```python
from build123d import *

# Parameters (mm, degrees)
CYLINDER013_R                      = 2.5
CYLINDER013_DEPTH                  = 19
CYLINDER012_R                      = 4.36
CYLINDER012_DEPTH                  = 5
FUSION001018017017_PLACEMENT_ANGLE = 180
POCKET002018_DEPTH                 = 2.5


with BuildPart() as cylinder013:
    # Cylinder013 → Cylinder013 (new body)
    with BuildSketch(Plane.XY):
        Circle(CYLINDER013_R)
    extrude(amount=CYLINDER013_DEPTH)


with BuildPart() as obj1:
    # Cylinder012 → Cylinder012 (new body)
    with BuildSketch(Plane.XY):
        Circle(CYLINDER012_R)
    extrude(amount=CYLINDER012_DEPTH)

    # Fusion001018017017: union Cylinder013
    add(cylinder013.part)


with BuildPart() as obj1_1:
    # Fusion001018017017 placement: moved
    add(obj1.part.rotate(Axis((0, 0, 0), (0, 1, 0)), FUSION001018017017_PLACEMENT_ANGLE))

    # Sketch019 → Pocket002018 (cut)
    with BuildSketch(Plane(origin=(0, 0, 0), x_dir=(-1, 0, 0), z_dir=(0, 0, 1))):
        Polygon((2, -1.154701), (2, 1.154701), (0, 2.309401), (-2, 1.154701), (-2, -1.154701), (0, -2.309401), align=None)
    extrude(amount=-POCKET002018_DEPTH, mode=Mode.SUBTRACT)


solid = obj1_1.part
```
Can you work these out from the model? Positions are in its coordinate system, mm. A direction names the side the tool comes from. Give positions to 0.01 mm unless a question says otherwise; leave off trailing zeros. Order: outer loops, then holes, each group sorted by start corner. A loop starts at its lowest first (then second) coordinate and runs counter-clockwise, first axis right, second up. Notation, with made-up numbers: (15.5, 88.5) - (61.5, 88.5) arc R11 cw to (61.5, 99.5) - close; hole circle Ø8 at (23, 31.5). An arc over 180 degrees is marked (long way). Use a Markdown table: item, result. Add a question column.
Q1. On a 3-axis mill with a long thin cutter (end or side, diameter ignored), from which of +Z, -Z, +X, -X, +Y, -Y can I reach the whole of each face in a straight line? I mean faces 1 (the flat face through (-2, -2, -5)), 2 (the flat face through (-0.99, 1.74, -1.23)), 3 (the cylindrical face through (0.945, -4.256, -2.465)). Say none if no direction works.
Q2. If we section it at B-B on y = 0: Write out the boundary of the cut face in (x, z).
Q3. If we section it at C-C on x = 1.5: Write out the boundary of the cut face in (y, z).
Q4. If we section it at A-A on z = -1.5: Write out the boundary of the cut face in (x, y), plus the area to 3 significant figures.
Q5. If we mould it in two halves opening along Y, with no side actions, what happens to faces 4 (the cylindrical face through (0.54, -2.44, -11.9)), 5 (the flat face through (-1, -2, 0)), 6 (the flat face through (-1.014, -1.724, -1.232))? For each: released by +Y, released by -Y, zero draft, split by the parting line, or undercut.
Q6. I'm going to push flat-ended pins straight in: pin 1 (2 mm diameter, centred on x = 0.5, y = 1, fed in from +Z); pin 2 (5 mm diameter, centred on y = -0.5, z = -15, fed in from +X); pin 3 (1.5 mm diameter, centred on y = -2, z = -3, fed in from -X); pin 4 (5 mm diameter, centred on y = -3, z = -12, fed in from +X). Where does each tip first touch, or does it pass through?
Q7. Please list where these lines run through material, in increasing order: line 1 along Z through (x, y) = (2.5, -3); line 2 along Z through (x, y) = (-0.75, -1); line 3 along X through (y, z) = (0, -7.25).
Q8. If we section it at D-D on z = -8.5: Write out the boundary of the cut face in (x, y), plus the area to 3 significant figures.
Answers follow:
| question | item | result |
|---|---|---|
| 1 | face 1 | -Z |
| 1 | face 2 | +Z |
| 1 | face 3 | +Z, -Z |
| 2 | outline | (-4.36, -5) - (-2.5, -5) - (-2.5, -19) - (2.5, -19) - (2.5, -5) - (4.36, -5) - (4.36, 0) - (2, 0) - (2, -2.5) - (-2, -2.5) - (-2, 0) - (-4.36, 0) - close |
| 3 | outline | (-4.09, -5) - (-2, -5) - (-2, -19) - (2, -19) - (2, -5) - (4.09, -5) - (4.09, 0) - (1.44, 0) - (1.44, -2.5) - (-1.44, -2.5) - (-1.44, 0) - (-4.09, 0) - close |
| 4 | outline | circle Ø8.72 at (0, 0); hole (-2, -1.15) - (0, -2.31) - (2, -1.15) - (2, 1.15) - (0, 2.31) - (-2, 1.15) - close |
| 4 | area | 45.9 mm^2 |
| 5 | face 4 | split by the parting line |
| 5 | face 5 | zero draft |
| 5 | face 6 | undercut |
| 6 | pin 1 | stops at z = 0 |
| 6 | pin 2 | stops at x = 2.5 |
| 6 | pin 3 | stops at x = -4.18 |
| 6 | pin 4 | stops at x = 2.45 |
| 7 | line 1 | z = -5 to 0 |
| 7 | line 2 | z = -19 to -2.5 |
| 7 | line 3 | x = -2.5 to 2.5 |
| 8 | outline | circle Ø5 at (0, 0) |
| 8 | area | 19.6 mm^2 |
